Verification items for the finished model (mm, model axes). Round coordinates to 2 decimals unless told otherwise and drop trailing zeros. One line per item, written item: value.
from build123d import *

# Parameters (mm, degrees)
SKETCH1_W           = 3302
SKETCH1_H           = 5461
SKETCH1_R           = 254
SKETCH1_R_2         = 127
SKETCH1_R_3         = 101.6
SKETCH1_R_4         = 63.5
BOSS_EXTRUDE1_DEPTH = 50
SCALE1_SCALE        = 0.04


with BuildPart() as part:
    # Sketch1 → Boss-Extrude1 (new body)
    with BuildSketch(Plane.XY):
        with Locations((1651, 2730.5)):
            Rectangle(SKETCH1_W, SKETCH1_H)
        with Locations((1873.2539878, 4935.236460216)):
            Circle(SKETCH1_R, mode=Mode.SUBTRACT)
        with Locations((603.2539878, 4935.236460216)):
            Circle(SKETCH1_R_2, mode=Mode.SUBTRACT)
        with Locations((603.2539878, 4300.236460216)):
            Circle(SKETCH1_R_3, mode=Mode.SUBTRACT)
        with Locations((603.2539878, 3665.236460216)):
            Circle(SKETCH1_R_4, mode=Mode.SUBTRACT)
        with Locations((1111.2539878, 4935.236460216)):
            Circle(SKETCH1_R_2, mode=Mode.SUBTRACT)
        with Locations((1111.2539878, 4300.236460216)):
            Circle(SKETCH1_R_3, mode=Mode.SUBTRACT)
        with Locations((1111.2539878, 3665.236460216)):
            Circle(SKETCH1_R_4, mode=Mode.SUBTRACT)
        with Locations((1873.2539878, 4300.236460216)):
            Circle(SKETCH1_R_3, mode=Mode.SUBTRACT)
        with Locations((1873.2539878, 3665.236460216)):
            Circle(SKETCH1_R_4, mode=Mode.SUBTRACT)
    extrude(amount=BOSS_EXTRUDE1_DEPTH)


with BuildPart() as part_1:
    # Scale1: scaled about (1656.511334765, 2681.700048918, 25)
    add(part.part.scale(SCALE1_SCALE).moved(Location((1590.250881374, 2574.432046961, 24))))


solid = part_1.part
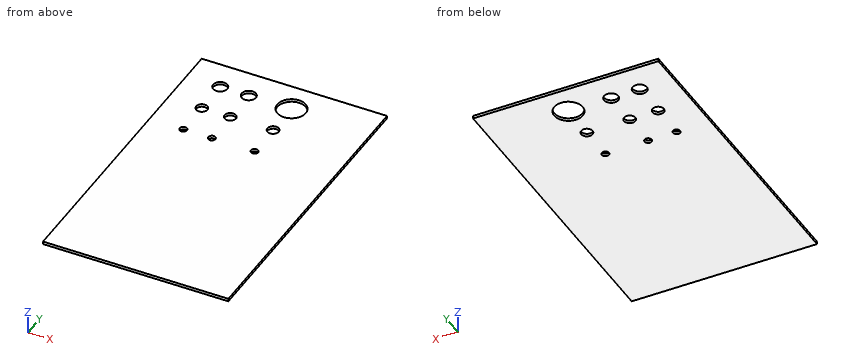
(1) Thickness scan on L1, parallel to X at y = 2746.5, z = 24.2; L2, parallel to X at y = 2771, z = 24.6; L3, parallel to X at y = 2762.5, z = 25.05. Record the ranges inside material, lowest first. Write a range as from..to.
Completed:
L1: x = 1590.25..1610.32, 1618.44..1630.64, 1638.76..1661.12, 1669.24..1722.33
L2: x = 1590.25..1609.37, 1619.39..1629.69, 1639.71..1655.06, 1675.31..1722.33
L3: x = 1590.25..1661.19, 1669.18..1722.33
(2) Sectioned sample at A-A on z = 25. Count the separate pieces of the cut face and the enclosed holes in it, and give its area (3 significant figures).
Completed:
separate pieces: 1
enclosed holes: 9
area: 28,100 mm^2
(3) Depth check by flat-ended pin: pin 1 Ø13 at (x, y) = (1665.18, 2746.44) entering from -Z; pin 2 Ø6.5 at (x, y) = (1634.7, 2746.44) entering from -Z (3 decimals). Enter the tip coordinate at first touch or a pass-through.
Completed:
pin 1: stops at z = 24
pin 2: passes through
